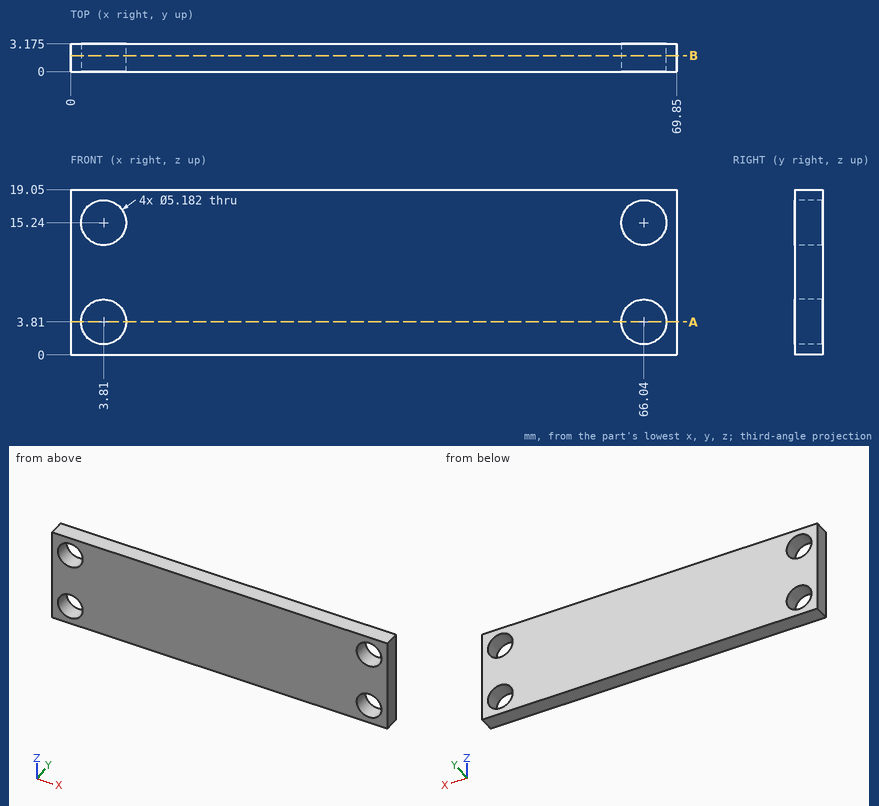
Input: dimensioned drawing with shaded views. Units: mm. Origin: part minimum x, y, z. Round coordinates to 2 decimals unless told otherwise and drop trailing zeros. Loops run counter-clockwise (first coordinate to the right, second up) from the corner with the lowest first, then second, coordinate; pieces in that order, holes last. Notation, with made-up numbers: (-35.75, 50.5) -> (3.25, 50.5) arc R27 cw to (3.25, 79.5) -> close; hole circle Ø4 at (23.25, -20). An arc over 180 degrees is marked (long way). One line per item, written item: value.
(1) Section B-B (y = 1.85). Return the cut outline in (x, z), plus the area to 3 significant figures.
Geometry check:
outline: (0, 0) -> (69.85, 0) -> (69.85, 19.05) -> (0, 19.05) -> close; hole circle Ø5.18 at (3.81, 3.81); hole circle Ø5.18 at (3.81, 15.24); hole circle Ø5.18 at (66.04, 3.81); hole circle Ø5.18 at (66.04, 15.24)
area: 1,250 mm2
(2) Section A-A (z = 3.81). Give the number of separate pieces and of enclosed holes in the cut face, plus the area to 3 significant figures.
Geometry check:
separate pieces: 3
enclosed holes: 0
area: 189 mm2
(3) Pin query (flat end, axial travel): pin 1 (6.5 mm diameter, centred on x = 66.04, z = 3.81, fed in from +Y) (3 decimals). Return the tip coordinate at first contact, or that it passes through.
Geometry check:
pin 1: y = 3.175
(4) Material intervals for line 1 (X direction, y = 2.35, z = 15.24); line 2 (Z direction, x = 3.81, y = 2.3); line 3 (X direction, y = 1.85, z = 4.5), sorted ascending. Write a range as [from, to].
Geometry check:
line 1: [0, 1.22], [6.4, 63.45], [68.63, 69.85]
line 2: [0, 1.22], [6.4, 12.65], [17.83, 19.05]
line 3: [0, 1.31], [6.31, 63.54], [68.54, 69.85]
